Autodesk Inventor part; units mm, degrees
ref_plane "YZ Plane" through (0, 0, 0) normal (1, 0, 0) x (0, 1, 0)
ref_plane "XZ Plane" through (0, 0, 0) normal (0, 1, 0) x (-1, 0, 0)
ref_plane "XY Plane" through (0, 0, 0) normal (0, 0, 1) x (1, 0, 0)
sketch "Sketch1" plane through (0, 0, 0) normal (0, 0, 1) x (1, 0, 0)
  line L0 (-102.5157, 69.2842) -> (97.4843, 69.2842)
  line L1 (97.4843, 69.2842) -> (97.4843, -80.7158)
  line L2 (97.4843, -80.7158) -> (-102.5157, -80.7158)
  line L3 (-102.5157, -80.7158) -> (-102.5157, 69.2842)
  point P0 (0, 0)
extrude "Extrusion1" add sketch "Sketch1" along normal blind 3
sketch "Sketch3" plane through (0, 0, 3) normal (0, 0, 1) x (1, 0, 0)
  point P0 (0, 0)
sketch "Sketch4" plane through (0, 0, 3) normal (0, 0, 1) x (1, 0, 0)
  line L0 (97.4843, 69.2842) -> (-102.5157, 69.2842)
  line L1 (-102.5157, 69.2842) -> (-99.5157, 69.2842)
  line L2 (-99.5157, 69.2842) -> (-99.5157, 19.2842)
  line L3 (-99.5157, 19.2842) -> (-102.5157, 19.2842)
  line L4 (-102.5157, 19.2842) -> (-102.5157, 69.2842)
  point P0 (0, 0)
extrude "Extrusion2" cut sketch "Sketch4" against normal blind 3
sketch "Sketch5" plane through (0, 0, 3) normal (0, 0, 1) x (1, 0, 0)
  line L0 (97.4843, -80.7158) -> (94.4843, -80.7158)
  line L1 (94.4843, -80.7158) -> (94.4843, -30.7158)
  line L2 (94.4843, -30.7158) -> (97.4843, -30.7158)
  line L3 (97.4843, -30.7158) -> (97.4843, -80.7158)
  point P0 (0, 0)
  point P1 (-102.5157, -80.7158)
  dimension "d17" = 3
  dimension "d18" = 50
extrude "Extrusion3" cut sketch "Sketch5" against normal blind 3
sketch "Sketch6" plane through (0, 0, 3) normal (0, 0, 1) x (1, 0, 0)
  line L0 (97.4843, -30.7158) -> (97.4843, 69.2842)
  line L1 (97.4843, 69.2842) -> (94.4843, 69.2842)
  line L2 (94.4843, 69.2842) -> (94.4843, 19.2842)
  line L3 (94.4843, 19.2842) -> (97.4843, 19.2842)
  line L4 (97.4843, 19.2842) -> (97.4843, 69.2842)
  point P0 (0, 0)
  dimension "d21" = 50
  dimension "d22" = 3
extrude "Extrusion4" cut sketch "Sketch6" against normal blind 3
sketch "Sketch7" plane through (0, 0, 3) normal (0, 0, 1) x (1, 0, 0)
  line L0 (-102.5157, 19.2842) -> (-102.5157, -80.7158)
  line L1 (-102.5157, -80.7158) -> (-99.5157, -80.7158)
  line L2 (-99.5157, -80.7158) -> (-99.5157, -30.7158)
  line L3 (-99.5157, -30.7158) -> (-102.5157, -30.7158)
  line L4 (-102.5157, -30.7158) -> (-102.5157, -80.7158)
  point P0 (0, 0)
  dimension "d25" = 50
  dimension "d26" = 3
extrude "Extrusion5" cut sketch "Sketch7" against normal blind 3
sketch "Sketch8" plane through (0, 0, 3) normal (0, 0, 1) x (1, 0, 0)
  line L0 (-102.5157, -30.7158) -> (-102.5157, 19.2842)
  line L1 (97.4843, -30.7158) -> (94.4843, -30.7158)
  line L2 (94.4843, -80.7158) -> (-99.5157, -80.7158)
  line L3 (-10.0157, -50.7158) -> (4.9843, -50.7158)
  line L4 (4.9843, -50.7158) -> (4.9843, -80.7158)
  line L5 (4.9843, -80.7158) -> (-10.0157, -80.7158)
  line L6 (-10.0157, -80.7158) -> (-10.0157, -50.7158)
  point P0 (0, 0)
  dimension "d32" = 15
  dimension "d33" = 30
extrude "Extrusion6" cut sketch "Sketch8" against normal blind 3
sketch "Sketch9" plane through (-10.0157, -80.7158, 3) normal (1, 0, 0) x (0, 0, -1)
  point P0 (3, 80.7158)
sketch "Sketch10" plane through (-10.0157, -50.7158, 3) normal (0, -1, 0) x (1, 0, 0)
  line L0 (15, 0) -> (15, -3)
  line L1 (15, -3) -> (0, -3)
  line L2 (15, 0) -> (0, 0)
  line L3 (0, 0) -> (0, -3)
  line L4 (0, -3) -> (15, -3)
  line L5 (15, -3) -> (15, 0)
  point P0 (10.0157, -3)
extrude "Extrusion7" add sketch "Sketch10" along normal blind 30
sketch "Sketch11" plane through (0, 0, 3) normal (0, 0, 1) x (1, 0, 0)
  line L0 (-102.5157, 19.2842) -> (-99.5157, 19.2842)
  line L1 (-99.5157, 69.2842) -> (94.4843, 69.2842)
  line L2 (94.4843, -80.7158) -> (-99.5157, -80.7158)
  line L3 (-99.5157, 19.2842) -> (-99.5157, 69.2842)
  line L4 (-102.5157, -30.7158) -> (-102.5157, 19.2842)
  line L5 (-2.5157, 9.2842) -> (-27.5157, 9.2842)
  line L6 (-2.5157, 9.2842) -> (-2.5157, -20.7158)
  line L7 (-27.5157, 9.2842) -> (-27.5157, -20.7158)
  line L8 (-2.5157, -20.7158) -> (-27.5157, -20.7158)
  circle A0 centre (4.9843, 1.9042) radius 2
  circle A1 centre (4.9843, -13.3358) radius 2
  point P0 (0, 0)
extrude "Extrusion8" cut sketch "Sketch11" against normal blind 21.5
sketch "Sketch12" plane through (0, 0, 3) normal (0, 0, 1) x (1, 0, 0)
  point P0 (0, 0)
sketch "Sketch13" plane through (0, 0, 3) normal (0, 0, 1) x (1, 0, 0)
  point P0 (0, 0)
sketch "Sketch14" plane through (0, 0, 3) normal (0, 0, 1) x (1, 0, 0)
  line L0 (97.4843, 19.2842) -> (97.4843, -30.7158)
  line L1 (-2.5157, -20.7158) -> (-2.5157, 9.2842)
  line L2 (36.2282, 8.4721) -> (58.5282, 8.4721)
  line L3 (58.5282, 8.4721) -> (58.5282, -19.8279)
  line L4 (58.5282, -19.8279) -> (36.2282, -19.8279)
  line L5 (36.2282, -19.8279) -> (36.2282, 8.4721)
  line L6 (-99.5157, 69.2842) -> (94.4843, 69.2842)
  point P0 (0, 0)
extrude "Extrusion9" cut sketch "Sketch14" against normal blind 30
sketch "Sketch15" plane through (0, 0, 3) normal (0, 0, 1) x (1, 0, 0)
  line L0 (36.2282, -19.8279) -> (36.2282, 8.4721)
  line L1 (36.2282, -19.8279) -> (58.5282, -19.8279)
  line L2 (36.2282, 8.4721) -> (58.5282, 8.4721)
  line L3 (58.5282, 8.4721) -> (58.5282, -19.8279)
  line L4 (58.5282, -19.8279) -> (36.2282, -19.8279)
  line L5 (36.2282, -19.8279) -> (36.2282, 8.4721)
  point P0 (0, 0)
extrude "Extrusion10" add sketch "Sketch15" against normal blind 3
sketch "Sketch16" plane through (0, 0, 3) normal (0, 0, 1) x (1, 0, 0)
  line L0 (-102.5157, -30.7158) -> (-102.5157, 19.2842)
  line L1 (97.4843, 19.2842) -> (97.4843, -30.7158)
  line L2 (-99.5157, 69.2842) -> (94.4843, 69.2842)
  line L3 (40.9489, 4.2992) -> (53.9459, 4.2992)
  line L4 (53.9459, 4.2992) -> (53.9459, -15.7008)
  line L5 (53.9459, -15.7008) -> (40.9489, -15.7008)
  line L6 (40.9489, -15.7008) -> (40.9489, 4.2992)
  point P0 (0, 0)
extrude "Extrusion11" cut sketch "Sketch16" against normal blind 3
sketch "Sketch17" plane through (0, 0, 3) normal (0, 0, 1) x (1, 0, 0)
  line L0 (40.9489, -15.7008) -> (40.9489, 4.2992)
  line L1 (-102.5157, -30.7158) -> (-102.5157, 19.2842)
  line L2 (53.9459, -15.7008) -> (53.9459, 4.2992)
  line L3 (97.4843, 19.2842) -> (97.4843, -30.7158)
  line L4 (40.9489, 4.2992) -> (53.9459, 4.2992)
  line L5 (53.9459, 4.2992) -> (53.9459, -15.7008)
  line L6 (53.9459, -15.7008) -> (40.9489, -15.7008)
  line L7 (40.9489, -15.7008) -> (40.9489, 4.2992)
  point P0 (0, 0)
extrude "Extrusion12" add sketch "Sketch17" against normal blind 3
sketch "Sketch18" plane through (0, 0, 3) normal (0, 0, 1) x (1, 0, 0)
  line L0 (97.4843, 19.2842) -> (97.4843, -30.7158)
  line L1 (-102.5157, -30.7158) -> (-102.5157, 19.2842)
  line L2 (-84.5157, 4.2842) -> (-71.5157, 4.2842)
  line L3 (-84.5157, 4.2842) -> (-71.5157, 4.2842)
  line L4 (-71.5157, 4.2842) -> (-71.5157, -15.7158)
  line L5 (-71.5157, -15.7158) -> (-84.5157, -15.7158)
  line L6 (-84.5157, -15.7158) -> (-84.5157, 4.2842)
  line L7 (79.4843, 4.2842) -> (66.4843, 4.2842)
  line L8 (79.4843, 4.2842) -> (66.4843, 4.2842)
  line L9 (66.4843, 4.2842) -> (66.4843, -15.7158)
  line L10 (66.4843, -15.7158) -> (79.4843, -15.7158)
  line L11 (79.4843, -15.7158) -> (79.4843, 4.2842)
  point P0 (0, 0)
extrude "Extrusion13" cut sketch "Sketch18" against normal blind 3
sketch "Sketch19" plane through (0, 0, 3) normal (0, 0, 1) x (1, 0, 0)
  point P0 (0, 0)
sketch "Sketch20" plane through (0, 0, 3) normal (0, 0, 1) x (1, 0, 0)
  line L0 (-84.5157, 4.2842) -> (-84.5157, -15.7158)
  line L1 (-71.5157, -15.7158) -> (-71.5157, 4.2842)
  line L2 (-84.5157, 4.2842) -> (-71.5157, 4.2842)
  line L3 (-71.5157, 4.2842) -> (-71.5157, -15.7158)
  line L4 (-71.5157, -15.7158) -> (-84.5157, -15.7158)
  line L5 (-84.5157, -15.7158) -> (-84.5157, 4.2842)
  point P0 (0, 0)
  dimension "d102" = 13
  dimension "d103" = 20
properties part number "Level1"
Part model, mm, in its own coordinate system. Give positions to 0.01 mm unless a question says otherwise; leave off trailing zeros. Order: outer loops, then holes, each group sorted by start corner. A loop starts at its lowest first (then second) coordinate and runs counter-clockwise, first axis right, second up. Notation, with made-up numbers: M 50.25,31.5 L 73.25,31.5 A17 ccw 73.25,46.5 Z; hole C 57.5,68 d4. An arc over 180 degrees is marked long. Use a Markdown table: item, result. Add a question column.
(1) Drop flat-ended pins along their axis: P1, Ø1.5, axis at x = -101, z = 1, coming from the +Y side; P2, Ø1.5, axis at x = -101, z = 1.5, coming from the -Y side. Give the stop position or say it passes through.
(2) Probe line 1 along Y through (x, z) = (74.5, 0.6); line 2 along X through (y, z) = (1.5, 2.6); line 3 along X through (y, z) = (3, 1.75). List the from-to ranges inside material, lowest first. Write a range as [from, to].
(3) Saw through at C-C, the plane z = 1.45. Give the cut face in (x, y), and give its area (3 significant figures).
(4) Mould opens along X. For faces 1 (the face through (-4, 12, 3)), 2 (the face through (6.892, -12.735, 1.521)) say: +X half, -X half, draft (parallel to the pull), parting line (faces both ways), or undercut.
(5) Saw through at A-A, the plane x = -19. Give the cut face in (y, z).
(6) Saw through at B-B, the plane y = -51. Give the cut face in (x, z), and give its area (3 significant figures).
Answer key:
| question | item | result |
|---|---|---|
| 1 | P1 | y = 19.28 |
| 1 | P2 | y = -30.72 |
| 2 | line 1 | [-80.72, -15.72], [4.28, 69.28] |
| 2 | line 2 | [-102.52, -84.52], [-71.52, -27.52], [-2.52, 3.03], [6.94, 66.48], [79.48, 97.48] |
| 2 | line 3 | [-102.52, -84.52], [-71.52, -27.52], [-2.52, 3.31], [6.66, 66.48], [79.48, 97.48] |
| 3 | outline | M -102.52,-30.72 L -99.52,-30.72 L -99.52,-80.72 L 94.48,-80.72 L 94.48,-30.72 L 97.48,-30.72 L 97.48,19.28 L 94.48,19.28 L 94.48,69.28 L -99.52,69.28 L -99.52,19.28 L -102.52,19.28 Z; hole M -84.52,-15.72 L -71.52,-15.72 L -71.52,4.28 L -84.52,4.28 Z; hole M -27.52,-20.72 L -2.52,-20.72 L -2.52,9.28 L -27.52,9.28 Z; hole C 4.98,-13.34 d4; hole C 4.98,1.9 d4; hole M 66.48,-15.72 L 79.48,-15.72 L 79.48,4.28 L 66.48,4.28 Z |
| 3 | area | 28,100 mm^2 |
| 4 | face 1 | draft |
| 4 | face 2 | undercut |
| 5 | outline | M -80.72,0 L -20.72,0 L -20.72,3 L -80.72,3 Z; M 9.28,0 L 69.28,0 L 69.28,3 L 9.28,3 Z |
| 6 | outline | M -99.52,0 L 94.48,0 L 94.48,3 L -99.52,3 Z |
| 6 | area | 582 mm^2 |
